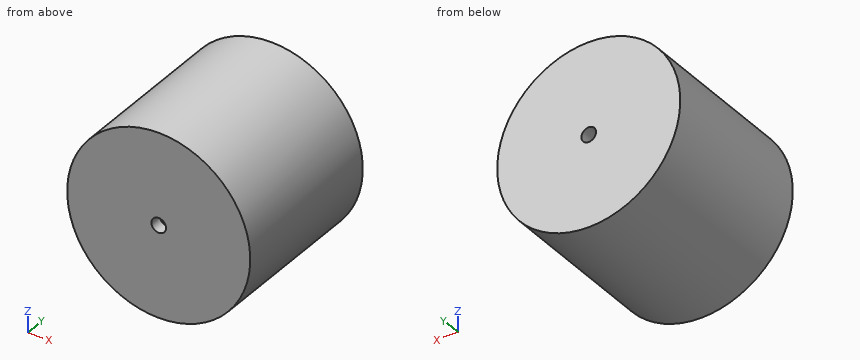
```python
from build123d import *

# Parameters (mm, degrees)
SKETCH1_R           = 75
SKETCH1_R_2         = 6
BOSS_EXTRUDE1_DEPTH = 135.4
SKETCH3_R           = 65
CUT_EXTRUDE2_DEPTH  = 110
SKETCH4_R           = 75
SKETCH4_R_2         = 6
BOSS_EXTRUDE2_DEPTH = 10


with BuildPart() as part:
    # Sketch1 → Boss-Extrude1 (new body)
    with BuildSketch(Plane(origin=(0, 0, 0), x_dir=(1, 0, 0), z_dir=(0, 1, 0))):
        with Locations(Location((0, 0, 0), (0, 0, 270))):
            Circle(SKETCH1_R)
        with Locations(Location((0, 0, 0), (0, 0, 270))):
            Circle(SKETCH1_R_2, mode=Mode.SUBTRACT)
    extrude(amount=BOSS_EXTRUDE1_DEPTH)

    # Sketch3 → Cut-Extrude2 (cut)
    with BuildSketch(Plane.XZ):
        with Locations(Location((0, 0, 0), (0, 0, 270))):
            Circle(SKETCH3_R)
    extrude(amount=-CUT_EXTRUDE2_DEPTH, mode=Mode.SUBTRACT)

    # Sketch4 → Boss-Extrude2 (add)
    with BuildSketch(Plane.XZ):
        with Locations(Location((0, 0, 0), (0, 0, 90))):
            Circle(SKETCH4_R)
        with Locations(Location((0, 0, 0), (0, 0, 270))):
            Circle(SKETCH4_R_2, mode=Mode.SUBTRACT)
    extrude(amount=-BOSS_EXTRUDE2_DEPTH)


solid = part.part
```
Design review of the part built by this model. Coordinates are the model's own, in mm. Round coordinates to 2 decimals unless told otherwise and drop trailing zeros. Order: outer loops, then holes, each group sorted by start corner. A loop starts at its lowest first (then second) coordinate and runs counter-clockwise, first axis right, second up. Notation, with made-up numbers: (-34, -40) - (2, -40) arc R9 cw to (2, -24) - close; hole circle Ø8 at (30.25, -8.5). An arc over 180 degrees is marked (long way). Return JSON: item names as keys, results as strings.
Q1. Consider section C-C on y = 15. Write out the cut boundary in (x, z), plus the area to 3 significant figures.
Computed values:
{"outline": "circle Ø150 at (0, 0); hole circle Ø130 at (0, 0)", "area": "4,400 mm2"}
Q2. For pin 1 Ø8 at (x, y) = (22, 69) entering from -Z; pin 2 Ø8 at (x, y) = (-40, 108.5) entering from -Z; pin 3 Ø5 at (y, z) = (68.5, -23.5) entering from -X; pin 4 Ø15.5 at (x, z) = (0, 0) entering from -Y, all flat-tipped, find the tip position at first contact; note any pin that passes through.
Computed values:
{"pin 1": "stops at z = -72.81", "pin 2": "stops at z = -65.8", "pin 3": "stops at x = -72", "pin 4": "stops at y = 0"}
Q3. Consider section A-A on x = 0. Write out the cut boundary in (y, z).
Computed values:
{"outline": "(0, -75) - (135.4, -75) - (135.4, -6) - (110, -6) - (110, -65) - (10, -65) - (10, -6) - (0, -6) - close; (0, 6) - (10, 6) - (10, 65) - (110, 65) - (110, 6) - (135.4, 6) - (135.4, 75) - (0, 75) - close"}
Q4. Consider section D-D on x = -43. Write out the cut boundary in (y, z).
Computed values:
{"outline": "(0, -61.45) - (135.4, -61.45) - (135.4, 61.45) - (0, 61.45) - close; hole (10, -48.74) - (110, -48.74) - (110, 48.74) - (10, 48.74) - close"}
Q5. Wall thickness on L1, parallel to X at y = 2, z = 0; L2, parallel to X at y = 70, z = 0; L3, parallel to Y at x = -8.5, z = -56: over which ranges is each line inside the solid? List them lowest first. Write a range as [from, to].
Computed values:
{"L1": "x = [-75, -6], [6, 75]", "L2": "x = [-75, -65], [65, 75]", "L3": "y = [0, 10], [110, 135.4]"}
Q6. Consider section B-B on z = 0. Write out the cut boundary in (x, y), plus the area to 3 significant figures.
Computed values:
{"outline": "(-75, 0) - (-6, 0) - (-6, 10) - (-65, 10) - (-65, 110) - (-6, 110) - (-6, 135.4) - (-75, 135.4) - close; (6, 0) - (75, 0) - (75, 135.4) - (6, 135.4) - (6, 110) - (65, 110) - (65, 10) - (6, 10) - close", "area": "6,890 mm2"}
